The listing builds one solid part. Answer for the finished solid, in the listing's coordinates (mm). A direction names the side the tool comes from. Round coordinates to 2 decimals unless told otherwise and drop trailing zeros. Order: outer loops, then holes, each group sorted by start corner. A loop starts at its lowest first (then second) coordinate and runs counter-clockwise, first axis right, second up. Notation, with made-up numbers: (29, -7) - (71, -7) arc R22 ccw to (71, 13) - close; hole circle Ø2 at (-36.5, -39.75). An arc over 180 degrees is marked (long way). Write item = value, one per line.
from build123d import *

# Parameters (mm, degrees)
SKETCH_1_W          = 12.25
SKETCH_1_H          = 11.3
EXTRUDE_1_DEPTH     = 2.5
SKETCH_2_W          = 1.5
SKETCH_2_H          = 11.3
EXTRUDE_2_DEPTH     = 3.85
SKETCH_5_W          = 9.25
SKETCH_5_H          = 11.5
CUT_EXTRUDE_1_DEPTH = 1
SKETCH_8_W          = 1.6
SKETCH_8_H          = 11.3
EXTRUDE_5_DEPTH     = 0.7
SKETCH_9_W          = 1.6
SKETCH_9_H          = 11.3
EXTRUDE_6_DEPTH     = 0.7
FILLET_8_R          = 0.3
SKETCH_11_W         = 12.25
SKETCH_11_H         = 4.85
CUT_EXTRUDE_2_DEPTH = 2
SKETCH_12_W         = 12.25
SKETCH_12_H         = 4.85
CUT_EXTRUDE_3_DEPTH = 2
SKETCH_13_W         = 1.5
SKETCH_13_H         = 11.3
EXTRUDE_7_DEPTH     = 0.5
SKETCH_14_W         = 1.5
SKETCH_14_H         = 11.3
EXTRUDE_8_DEPTH     = 0.5
FILLET_9_R          = 0.5
FILLET_10_R         = 0.7
FILLET_11_R         = 0.75


with BuildPart() as part:
    # 스케치1 → 보스-돌출1 (new body)
    with BuildSketch(Plane.XY):
        Rectangle(SKETCH_1_W, SKETCH_1_H)
    extrude(amount=EXTRUDE_1_DEPTH)

    # 스케치2 → 보스-돌출2 (add)
    with BuildSketch(Plane.XY.offset(2.5)):
        with Locations((-5.375, 0)):
            Rectangle(SKETCH_2_W, SKETCH_2_H)
        with Locations((5.375, 0)):
            Rectangle(SKETCH_2_W, SKETCH_2_H)
    extrude(amount=EXTRUDE_2_DEPTH)

    # 스케치5 → 컷-돌출1 (cut)
    with BuildSketch(Plane.XY.offset(2.5)):
        Rectangle(SKETCH_5_W, SKETCH_5_H)
    extrude(amount=-CUT_EXTRUDE_1_DEPTH, mode=Mode.SUBTRACT)

    # 스케치8 → 보스-돌출5 (add)
    with BuildSketch(Plane(origin=(-4.625, 0, 0), x_dir=(0, 0, -1), z_dir=(1, 0, 0))):
        with Locations((-5.55, 0)):
            Rectangle(SKETCH_8_W, SKETCH_8_H)
    extrude(amount=EXTRUDE_5_DEPTH)

    # 스케치9 → 보스-돌출6 (add)
    with BuildSketch(Plane.ZY.offset(-4.625)):
        with Locations((5.55, 0)):
            Rectangle(SKETCH_9_W, SKETCH_9_H)
    extrude(amount=EXTRUDE_6_DEPTH)

    # 필렛8
    fillet_8_edges = [part.edges().sort_by_distance(p)[0] for p in [
        (4.625, 0, 1.5),
        (-4.625, 0, 1.5),
    ]]
    fillet(fillet_8_edges, radius=FILLET_8_R)

    # 스케치11 → 컷-돌출2 (cut)
    with BuildSketch(Plane(origin=(0, 5.65, 0), x_dir=(1, 0, 0), z_dir=(0, 1, 0))):
        with Locations((0, -3.925)):
            Rectangle(SKETCH_11_W, SKETCH_11_H)
    extrude(amount=-CUT_EXTRUDE_2_DEPTH, mode=Mode.SUBTRACT)

    # 스케치12 → 컷-돌출3 (cut)
    with BuildSketch(Plane.XZ.offset(5.65)):
        with Locations((0, 3.925)):
            Rectangle(SKETCH_12_W, SKETCH_12_H)
    extrude(amount=-CUT_EXTRUDE_3_DEPTH, mode=Mode.SUBTRACT)

    # 스케치13 → 보스-돌출7 (add)
    with BuildSketch(Plane(origin=(6.125, 0, 0), x_dir=(0, 0, -1), z_dir=(1, 0, 0))):
        with Locations((-0.75, 0)):
            Rectangle(SKETCH_13_W, SKETCH_13_H)
    extrude(amount=EXTRUDE_7_DEPTH)

    # 스케치14 → 보스-돌출8 (add)
    with BuildSketch(Plane.ZY.offset(6.125)):
        with Locations((0.75, 0)):
            Rectangle(SKETCH_14_W, SKETCH_14_H)
    extrude(amount=EXTRUDE_8_DEPTH)

    # 필렛9
    fillet_9_edges = [part.edges().sort_by_distance(p)[0] for p in [
        (6.125, 0, 1.5),
        (-6.125, 0, 1.5),
    ]]
    fillet(fillet_9_edges, radius=FILLET_9_R - 0.0001)  # a hair under: the kernel refuses the full size

    # 필렛10
    fillet_10_edges = [part.edges().sort_by_distance(p)[0] for p in [
        (-3.925, 0, 6.35),
        (-3.925, 0, 4.75),
        (3.925, 0, 4.75),
        (3.925, 0, 6.35),
    ]]
    fillet(fillet_10_edges, radius=FILLET_10_R - 0.0001)  # a hair under: the kernel refuses the full size

    # 필렛11
    fillet_11_edges = [part.edges().sort_by_distance(p)[0] for p in [
        (6.625, -5.65, 0.75),
        (6.625, 5.65, 0.75),
        (-6.625, 5.65, 0.75),
        (-6.625, -5.65, 0.75),
    ]]
    fillet(fillet_11_edges, radius=FILLET_11_R)


solid = part.part
Q1. Section B-B on x = -5.5 is taken. Determine the outline of the cut face in (y, z), then the cut area to 3 significant figures.
Model answer:
outline = (-5.65, 0) - (5.65, 0) - (5.65, 1.5) - (3.65, 1.5) - (3.65, 6.35) - (-3.65, 6.35) - (-3.65, 1.5) - (-5.65, 1.5) - close
area = 52.4 mm^2
Q2. Determine the mould class of faces 1 (the face through (0, 0, 0)), 2 (the face through (-4.625, 0, 3)), 3 (the face through (-5, 0, 6.35)), 4 (the face through (5, -3.65, 4)) for opening direction Z: released by +Z, released by -Z, zero draft, split by the parting line, or undercut.
Model answer:
face_1 = released by -Z
face_2 = undercut
face_3 = released by +Z
face_4 = zero draft
Q3. Find the intervals of material crossed by line 1 (X direction, y = -3, z = 4.5) (3 decimals); line 2 (Y direction, x = 5.25, z = 2.5); line 3 (Z direction, x = -5.5, y = -4), in increasing order. Write a range as from..to.
Model answer:
line_1 = -6.125..-4.625, 4.625..6.125
line_2 = -3.65..3.65
line_3 = 0..1.5
Q4. Flat-ended cylindrical pins translate along their axes: P1, Ø0.8, axis at x = -5, z = 5, coming from the -Y side; P2, Ø2, axis at y = 1, z = 3, coming from the +X side (3 decimals); P3, Ø3, axis at y = 0.5, z = 3.5, coming from the -X side (3 decimals). Find the tip coordinate at first contact, or state that the pin passes through.
Model answer:
P1 = -3.65
P2 = 6.125
P3 = -6.125
Q5. Section D-D on x = 0.5 is taken. Determine the outline of the cut face in (y, z).
Model answer:
outline = (-5.65, 0) - (5.65, 0) - (5.65, 1.5) - (-5.65, 1.5) - close
Q6. For faces 5 (the face through (-5, -3.65, 4)), 6 (the face through (6.125, 0, 4)), 7 (the face through (-6.125, 0, 4)), 8 (the face through (4.625, 0, 3)), determine the directions among +Z, -Z, +X, -X, +Y, -Y from which every point of the face is accessible in a straight line to the end or side of a thin tool.
Model answer:
face_5 = +Z, +X, -X, -Y
face_6 = +Z, +X, +Y, -Y
face_7 = +Z, -X, +Y, -Y
face_8 = +Y, -Y
Q7. Section A-A on z = 2.25 is taken. Determine the outline of the cut face in (x, y) (3 decimals).
Model answer:
outline = (-6.125, -3.65) - (-4.625, -3.65) - (-4.625, 3.65) - (-6.125, 3.65) - close; (4.625, -3.65) - (6.125, -3.65) - (6.125, 3.65) - (4.625, 3.65) - close
